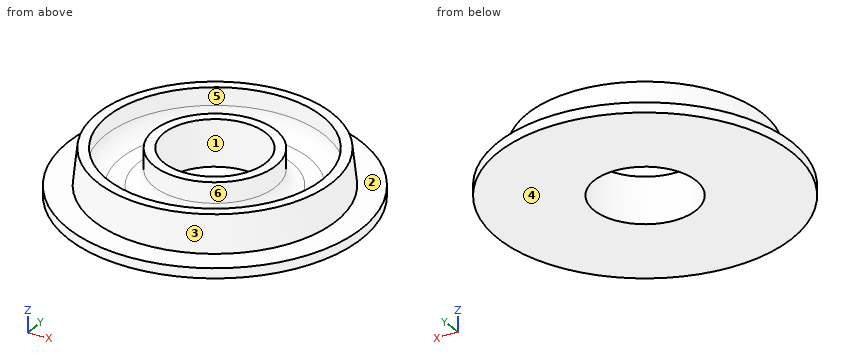
from build123d import *

# Parameters (mm, degrees)
F2_T = -3.175
F3_R = 5.08
F4_R = 5.08


with BuildPart() as f1:
    # F0 (on Front) → F1 (revolve)
    with BuildSketch(Plane.XZ):
        Polygon((-16.3068, 2.9675877146), (-16.3068, 17.7895731165), (-37.592, 17.7895731165), (-38.862, 6.1425877146), (-46.99, 6.1425877146), (-46.99, 2.9675877146), align=None)
    revolve(axis=Axis((0, 0, 15.8357990333), (0, 0, 1)))

    # F2
    f2_openings = [f1.faces().sort_by_distance(p)[0] for p in [
        (17.370062, 0, 17.789573),
    ]]
    offset(amount=F2_T, openings=f2_openings)

    # F3
    f3_edges = [f1.edges().sort_by_distance(p)[0] for p in [
        (19.4818, 0, 6.142588),
    ]]
    fillet(f3_edges, radius=F3_R)

    # F4
    f4_edges = [f1.edges().sort_by_distance(p)[0] for p in [
        (35.66818, 0, 6.142588),
    ]]
    fillet(f4_edges, radius=F4_R)


solid = f1.part
Read the model definition and answer for the solid it produces. Units are mm, in the model's axes. Face numbers are marked on the shaded views. A direction names the side the tool comes from. Round coordinates to 2 decimals unless told otherwise and drop trailing zeros. Loops run counter-clockwise (first coordinate to the right, second up) from the corner with the lowest first, then second, coordinate; pieces in that order, holes last. Notation, with made-up numbers: (60, 12.5) - (116, 12.5) arc R15 cw to (116, 33.5) - close; hole circle Ø8 at (-13, 71.25). An arc over 180 degrees is marked (long way). One line per question, with ' | ' between items. Start each with the question number.
Q1. Find the intervals of material crossed by L1, parallel to Y at x = -16.5, z = 7.75; L2, parallel to Y at x = 0, z = 11; L3, parallel to Y at x = 0, z = 10.5, in increasing order.
Q2. Flat-ended cylindrical pins translate along their axes: pin 1 (5 mm diameter, centred on y = -36.5, z = 9, fed in from +X); pin 2 (3 mm diameter, centred on y = -2, z = 5, fed in from +X); pin 3 (8 mm diameter, centred on y = -29, z = 10.5, fed in from -X). Find the tip coordinate at first contact, or state that the pin passes through.
Q3. Section C-C on z = 8.75 is taken. Give the vertices of the cut face in (x, y), plus the area to 3 significant figures.
Q4. For a pull along Y with two mould halves and no side action, classify the marked faces 1, 2 and 3 as +Y half, -Y half, draft (parallel to the pull), parting line (faces both ways), or undercut.
Q5. For the marked faces 4, 5 and 6, determine the directions among +Z, -Z, +X, -X, +Y, -Y from which every point of the face is accessible in a straight line to the end or side of a thin tool.
Q6. Section A-A on y = 0 is taken. Give the vertices of the cut face in (x, z).
Established:
1) L1: -34.99 to -29.4, -12.75 to 12.75, 29.4 to 34.99 | L2: -38.33 to -35.08, -19.49 to -16.31, 16.31 to 19.49, 35.08 to 38.33 | L3: -38.39 to -35.03, -19.53 to -16.31, 16.31 to 19.53, 35.03 to 38.39
2) pin 1: x = 18.21 | pin 2: x = 46.99 | pin 3: x = -29.18
3) outline: circle Ø77.16 at (0, 0); circle Ø40.25 at (0, 0); hole circle Ø68.88 at (0, 0); hole circle Ø32.61 at (0, 0) | area: 1,390 mm²
4) face 1: undercut | face 2: draft | face 3: parting line
5) face 4: -Z, +X, -X, +Y, -Y | face 5: none | face 6: +Z
6) outline: (-46.99, 2.97) - (-16.31, 2.97) - (-16.31, 17.79) - (-19.48, 17.79) - (-19.48, 11.22) arc R5.08 cw to (-24.56, 6.14) - (-30, 6.14) arc R5.08 cw to (-35.05, 11.77) - (-34.4, 17.79) - (-37.59, 17.79) - (-38.86, 6.14) - (-46.99, 6.14) - close; (16.31, 2.97) - (46.99, 2.97) - (46.99, 6.14) - (38.86, 6.14) - (37.59, 17.79) - (34.4, 17.79) - (35.05, 11.77) arc R5.08 cw to (30, 6.14) - (24.56, 6.14) arc R5.08 cw to (19.48, 11.22) - (19.48, 17.79) - (16.31, 17.79) - close
